For this review, use the dimensioned drawing (mm, ordinates from the lowest corner) and the shaded views. A direction names the side the tool comes from. Coordinates: 2 decimals unless noted, no trailing zeros. Write each loop counter-clockwise with the first axis right and the second up, starting at its lowest first coordinate (ties: lowest second). Pieces come first, ordered by that corner, then holes. Notation, with made-up numbers: M 40,77 L 50,77 A20 cw 50,101 Z; hole C 67.25,32.25 d9. An arc over 180 degrees is marked long. Return JSON: item names as keys, results as strings.
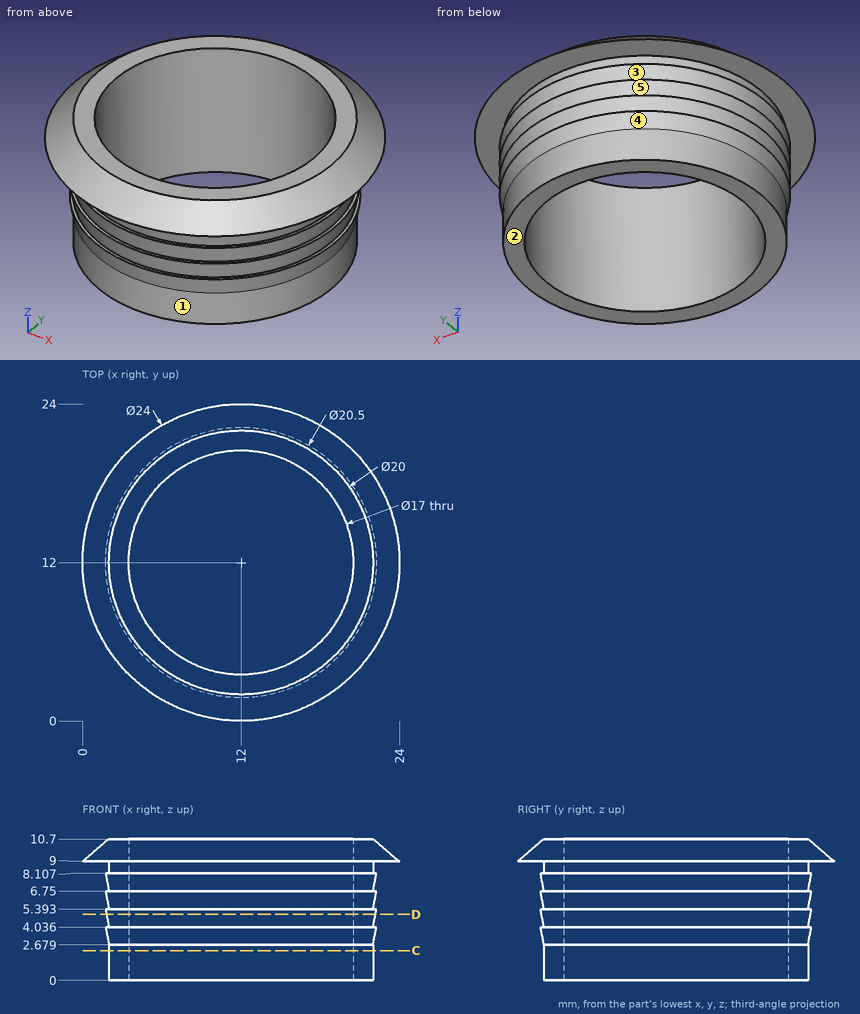
1. Draft analysis for pull direction Z (two halves, no side actions). For the marked faces 1, 2 and 3, state which applies: +Z half, -Z half, draft (parallel to the pull), parting line (faces both ways), or undercut.
Checks:
{"face 1": "draft", "face 2": "-Z half", "face 3": "undercut"}
2. For the marked faces 4 and 5, list the 3-axis set-ups (+Z, -Z, +X, -X, +Y, -Y) from which the entire face can be reached by the end or side of a thin tool; tool diameter is ignored.
Checks:
{"face 4": "-Z", "face 5": "none"}
3. Clearance check with flat-ended pins moving along their axes: pin 1 Ø1 at (x, z) = (18.5, 2) entering from -Y; pin 2 Ø1 at (y, z) = (9.5, 4) entering from +X. State where each tip first meets the part, or that it passes through.
Checks:
{"pin 1": "y = 4", "pin 2": "x = 22.05"}
4. We need section C-C (z = 2.25). State the section outline as (x, y) points.
Checks:
{"outline": "C 12,12 d20; hole C 12,12 d17"}
5. We need section D-D (z = 5). State the section outline as (x, y) points (1 decimal).
Checks:
{"outline": "C 12,12 d20.4; hole C 12,12 d17"}
6. Wall thickness on L1, parallel to Y at x = 12, z = 4; L2, parallel to Y at x = 12, z = 2.25; L3, parallel to X at y = 7.5, z = 9.5: over which ranges is each line inside the solid? List them lowest first. Write a range as from..to.
Checks:
{"L1": "1.76..3.5, 20.5..22.24", "L2": "2..3.5, 20.5..22", "L3": "1.51..4.79, 19.21..22.49"}
